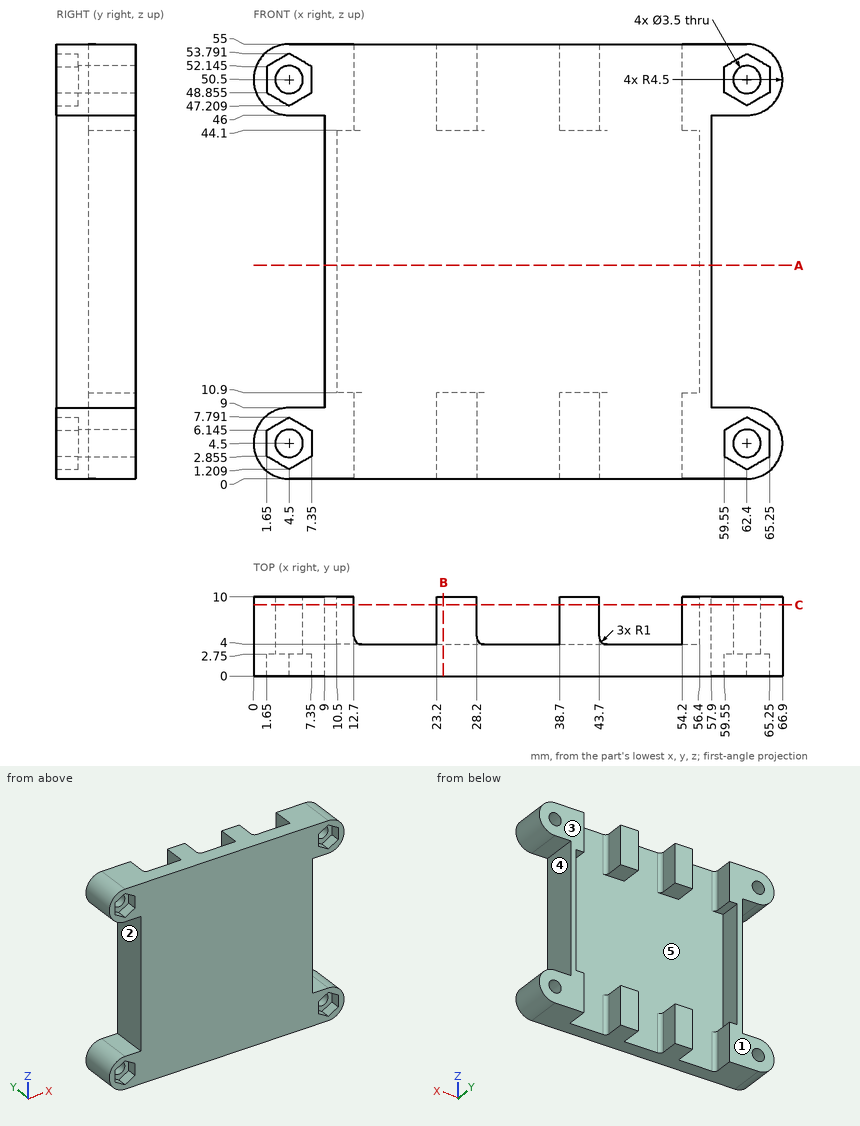
Geometry: see drawing. Coordinates: mm, zero at the bounding-box minimum. A direction names the side the tool comes from. Give positions to 0.01 mm unless a question says otherwise; leave off trailing zeros. Write each loop counter-clockwise with the first axis right and the second up, starting at its lowest first coordinate (ties: lowest second). Pieces come first, ordered by that corner, then holes. Notation, with made-up numbers: (83, 59.5) - (136, 59.5) arc R18 ccw to (136, 92.5) - close; hole circle Ø11 at (24.25, 63). An arc over 180 degrees is marked (long way). Return JSON: item names as keys, results as strings. Group by question number.
1) Line query: line 1 (X direction, y = 7.5, z = 26); line 2 (Z direction, x = 58, y = 1.5); line 3 (X direction, y = 8, z = 3) (1 decimal). Output: solid intervals per line, ascending.
2) Mould query, pull axis X, two halves, no side actions, for the marked faces 3, 4 and 5. Classes: released by +X, released by -X, zero draft, split by the parting line, or undercut.
3) Section B-B on x = 24. Return the cut outline in (y, z), plus the area to 3 significant figures.
4) First-contact query: P1, Ø2, axis at x = 28, z = 18.5, coming from the +Y side; P2, Ø5, axis at y = 8, z = 29.5, coming from the +X side; P3, Ø3, axis at y = 7, z = 9, coming from the -X side (1 decimal). Flat tips, straight axial feed; report the tip coordinate or a pass-through.
5) Set-up query: the marked faces 1 and 2. Return all of +Z, -Z, +X, -X, +Y, -Y with unobstructed straight access to the full face (end or side cutting, diameter ignored); none if empty.
6) Section C-C on y = 9. State how many separate pieces and enclosed holes the cut face has.
7) Section A-A on z = 27. Return the cut outline in (x, y).
Filled in:
{
 "1": {"line 1": "x = 9 to 10.5, 56.4 to 57.9", "line 2": "z = 0 to 9, 46 to 55", "line 3": "x = 0.3 to 3.6, 5.4 to 12.7, 23.2 to 28.2, 38.7 to 43.7, 54.2 to 61.5, 63.3 to 66.6"},
 "2": {"face 3": "zero draft", "face 4": "released by +X", "face 5": "undercut"},
 "3": {"outline": "(0, 0) - (10, 0) - (10, 10.9) - (4, 10.9) - (4, 44.1) - (10, 44.1) - (10, 55) - (0, 55) - close", "area": "351 mm^2"},
 "4": {"P1": "stops at y = 4", "P2": "stops at x = 57.9", "P3": "stops at x = 1.1"},
 "5": {"face 1": "+Z, -Z, +X, -X, +Y", "face 2": "-X, +Y, -Y"},
 "6": {"separate pieces": "6", "enclosed holes": "4"},
 "7": {"outline": "(9, 0) - (57.9, 0) - (57.9, 10) - (56.4, 10) - (56.4, 4) - (10.5, 4) - (10.5, 10) - (9, 10) - close"}
}
